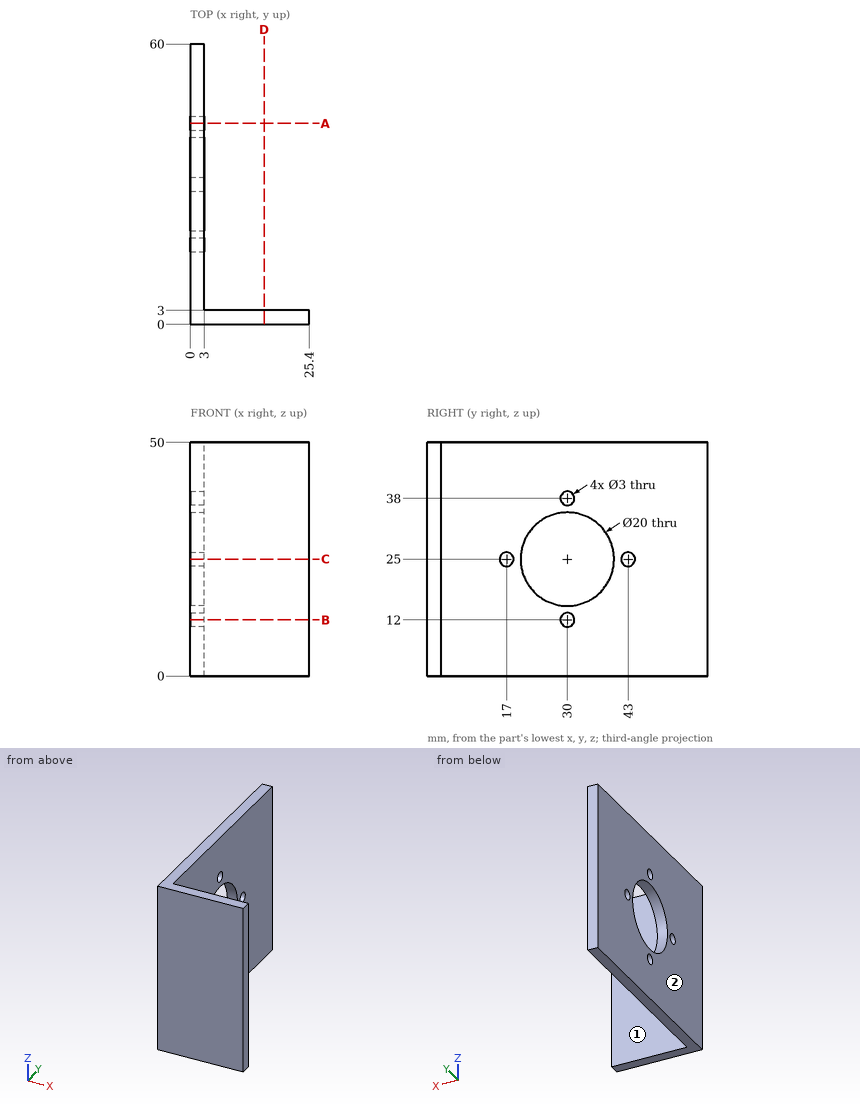
Design review of the part shown in the three views and the two pictorial views. Dimensions are in mm from the part's minimum x, y and z. A direction names the side the tool comes from. Round coordinates to 2 decimals unless told otherwise and drop trailing zeros. Loops run counter-clockwise (first coordinate to the right, second up) from the corner with the lowest first, then second, coordinate; pieces in that order, holes last. Notation, with made-up numbers: (-23, -5.75) -> (18, -5.75) arc R22 cw to (18, 6.25) -> close; hole circle Ø11 at (26, -17.5). An arc over 180 degrees is marked (long way). Answer as a JSON object with one key per item and string values. Group by question number.
1) We need section D-D on x = 15.75. Write out the cut boundary in (y, z), then the cut area to 3 significant figures.
2) For the marked faces 1 and 2, list the 3-axis set-ups (+Z, -Z, +X, -X, +Y, -Y) from which the entire face can be reached by the end or side of a thin tool; tool diameter is ignored.
3) For pin 1 Ø4 at (y, z) = (17, 25) entering from +X, flat-tipped, find the tip position at first contact; note if it passes through.
4) We need section A-A on y = 43. Write out the cut boundary in (x, z), then the cut area to 3 significant figures.
5) We need section C-C on z = 25. Write out the cut boundary in (x, y).
6) For line 1 (Y direction, x = 2.2, z = 25); line 2 (Y direction, x = 1.8, z = 12); line 3 (X direction, y = 19, z = 39.5), list the stretches that pass through material, from the lowest coordinate up. Write a range as [from, to].
7) We need section B-B on z = 12. Write out the cut boundary in (x, y), then the cut area to 3 significant figures.
Result set:
{
 "1": {"outline": "(0, 0) -> (3, 0) -> (3, 50) -> (0, 50) -> close", "area": "150 mm²"},
 "2": {"face 1": "+Z, -Z, +X, +Y", "face 2": "+Z, -Z, -X, +Y, -Y"},
 "3": {"pin 1": "x = 3"},
 "4": {"outline": "(0, 0) -> (3, 0) -> (3, 23.5) -> (0, 23.5) -> close; (0, 26.5) -> (3, 26.5) -> (3, 50) -> (0, 50) -> close", "area": "141 mm²"},
 "5": {"outline": "(0, 0) -> (25.4, 0) -> (25.4, 3) -> (3, 3) -> (3, 15.5) -> (0, 15.5) -> close; (0, 18.5) -> (3, 18.5) -> (3, 20) -> (0, 20) -> close; (0, 40) -> (3, 40) -> (3, 41.5) -> (0, 41.5) -> close; (0, 44.5) -> (3, 44.5) -> (3, 60) -> (0, 60) -> close"},
 "6": {"line 1": "[0, 15.5], [18.5, 20], [40, 41.5], [44.5, 60]", "line 2": "[0, 28.5], [31.5, 60]", "line 3": "[0, 3]"},
 "7": {"outline": "(0, 0) -> (25.4, 0) -> (25.4, 3) -> (3, 3) -> (3, 28.5) -> (0, 28.5) -> close; (0, 31.5) -> (3, 31.5) -> (3, 60) -> (0, 60) -> close", "area": "238 mm²"}
}
